Work out the finished part from the listing and answer in its coordinate system (mm). Face numbers are marked on the shaded views. A direction names the side the tool comes from. Give positions to 0.01 mm unless a question says otherwise; leave off trailing zeros. Write each loop counter-clockwise with the first axis right and the second up, starting at its lowest first coordinate (ties: lowest second). Pieces come first, ordered by that corner, then holes.
1) Determine the mould class of the marked faces 5, 6 and 7 for opening direction Z: pulls with the +Z half, pulls with the -Z half, needs draft (parallel to the pull), parting line crosses it, or undercut.
2) Find section B-B (y = 21). Determine the outline of the cut face in (x, z).
3) Given pin 1 Ø1 at (y, z) = (36, -4.5) entering from +X; pin 2 Ø12 at (y, z) = (18, 4) entering from -X; pin 3 Ø4 at (x, z) = (74.1, -1.7) entering from +Y; pin 4 Ø6.5 at (x, z) = (68.3, 21.5) entering from +Y, each flat-ended and moving along its own axis, determine where each tip first touches the part or whether it passes through.
4) Find section D-D (z = 16). Determine the outline of the cut face in (x, y).
5) A tool of negligible diameter and unlimited length cuts with its end or side. For the marked faces 1, 2, 3 and 4, from which of +Z, -Z, +X, -X, +Y, -Y can it reach the whole face along a straight path? Write none if from no direction.
6) Straight lines are drawn through the part: probe 1 along Z at (x, y) = (68, 23); probe 2 along Z at (x, y) = (-100, 9.75); probe 3 along Z at (x, y) = (-3.5, 8). For each, find the intervals that lie inside material, in ascending order.
7) Find section A-A (x = 74.1). Determine the outline of the cut face in (y, z), plus the area to 3 significant figures.
8) Find section C-C (x = 12). Determine the outline of the cut face in (y, z).
```python
from build123d import *
from build123d.topology import SkipClean

# Parameters (mm, degrees)
SKETCH1_W           = 195
SKETCH1_H           = 67
BOSS_EXTRUDE1_DEPTH = 50
CUT_EXTRUDE1_DEPTH  = 115.579666608
CUT_EXTRUDE2_DEPTH  = 129.433835106
CUT_EXTRUDE3_START  = -13
SKETCH4_W           = 3.612655346
SKETCH4_H           = 3
CUT_EXTRUDE3_DEPTH  = 13
SKETCH6_R           = 2.5
CUT_EXTRUDE4_DEPTH  = 115.579666608
SKETCH7_W           = 37
SKETCH7_H           = 35
CUT_EXTRUDE5_DEPTH  = 1.5
CUT_EXTRUDE6_DEPTH  = 18.5
SKETCH9_R           = 2.5
CUT_EXTRUDE7_DEPTH  = 25
BOSS_EXTRUDE2_START = 25
BOSS_EXTRUDE2_DEPTH = 25
BOSS_EXTRUDE3_DEPTH = 2


with BuildPart() as part:
    # Sketch1 → Boss-Extrude1 (new body)
    with BuildSketch(Plane(origin=(0, 0, 0), x_dir=(1, 0, 0), z_dir=(0, 1, 0))):
        Rectangle(SKETCH1_W, SKETCH1_H)
    extrude(amount=BOSS_EXTRUDE1_DEPTH)

    # Sketch2 → Cut-Extrude1 (cut, through all)
    with BuildSketch(Plane.XZ):
        with BuildLine():
            Line((97.5, -3.219751644), (97.5, 33.5))
            Line((97.5, 33.5), (88.5, 33.5))
            ThreePointArc((88.5, 33.5), (95.217186872, 15.683556008), (97.5, -3.219751644))
        make_face()
        with BuildLine():
            Line((97.5, -33.5), (97.5, -3.219751644))
            ThreePointArc((97.5, -3.219751644), (95.985558513, -18.65423771), (91.5, -33.5))
            Line((91.5, -33.5), (97.5, -33.5))
        make_face()
        with BuildLine():
            ThreePointArc((-88, -33.5), (-95.08607052, -15.861694529), (-97.5, 2.992884749))
            Line((-97.5, 2.992884749), (-97.5, -33.5))
            Line((-97.5, -33.5), (-88, -33.5))
        make_face()
        with BuildLine():
            ThreePointArc((-97.5, 2.992884749), (-95.856964648, 18.588830376), (-91, 33.5))
            Line((-91, 33.5), (-97.5, 33.5))
            Line((-97.5, 33.5), (-97.5, 2.992884749))
        make_face()
    extrude(amount=-CUT_EXTRUDE1_DEPTH, mode=Mode.SUBTRACT)

    # Sketch3 → Cut-Extrude2 (cut, through all)
    with BuildSketch(Plane(origin=(0, 0, 33.5), x_dir=(-1, 0, 0), z_dir=(0, 0, -1))):
        Polygon((63.2, 50), (63.2, 39.6), (40.2, 39.6), (40.2, 35.6), (-61.8, 35.6), (-61.8, 39.6), (-97.5, 39.6), (-97.5, 50), align=None)
    extrude(amount=CUT_EXTRUDE2_DEPTH, mode=Mode.SUBTRACT)

    # Sketch4 → Cut-Extrude3 (cut)
    with BuildSketch(Plane(origin=(0, 50, 0), x_dir=(1, 0, 0), z_dir=(0, 1, 0)).offset(CUT_EXTRUDE3_START)):
        with BuildLine():
            Line((-63.2, 30.5), (-63.2, 33.5))
            Line((-63.2, 33.5), (-88, 33.5))
            ThreePointArc((-88, 33.5), (-88.810680862, 32.008999469), (-89.587344654, 30.5))
            Line((-89.587344654, 30.5), (-63.2, 30.5))
        make_face()
        with Locations((-61.393672327, 32)):
            Rectangle(SKETCH4_W, SKETCH4_H)
        with BuildLine():
            Line((-63.2, -33.5), (-63.2, -30.5))
            Line((-63.2, -30.5), (-92.261692194, -30.5))
            ThreePointArc((-92.261692194, -30.5), (-91.647155152, -32.006859002), (-91, -33.5))
            Line((-91, -33.5), (-63.2, -33.5))
        make_face()
        with Locations((-61.393672327, -32)):
            Rectangle(SKETCH4_W, SKETCH4_H)
    extrude(amount=CUT_EXTRUDE3_DEPTH, mode=Mode.SUBTRACT)

    # Sketch6 → Cut-Extrude4 (cut, through all)
    with BuildSketch(Plane.XZ):
        with Locations(Location((-28.1, -9, 0), (0, 0, 270))):
            Circle(SKETCH6_R)
        with Locations(Location((-8.2, -8.3, 0), (0, 0, 270))):
            Circle(SKETCH6_R)
        with Locations(Location((-18.7, 8.7, 0), (0, 0, 270))):
            Circle(SKETCH6_R)
        with Locations(Location((-76.2, 22, 0), (0, 0, 270))):
            Circle(SKETCH6_R)
        with Locations(Location((-78.2, 0.1, 0), (0, 0, 270))):
            Circle(SKETCH6_R)
        with Locations(Location((-73.2, -22.3, 0), (0, 0, 270))):
            Circle(SKETCH6_R)
        with Locations(Location((65.3, -20, 0), (0, 0, 270))):
            Circle(SKETCH6_R)
        with Locations(Location((74.1, -1.7, 0), (0, 0, 270))):
            Circle(SKETCH6_R)
        with Locations(Location((68.3, 21.5, 0), (0, 0, 270))):
            Circle(SKETCH6_R)
    extrude(amount=-CUT_EXTRUDE4_DEPTH, mode=Mode.SUBTRACT)

    # Sketch7 → Cut-Extrude5 (cut)
    with BuildSketch(Plane(origin=(0, 35.6, 0), x_dir=(1, 0, 0), z_dir=(0, 1, 0))):
        with Locations((5.3, -16)):
            Rectangle(SKETCH7_W, SKETCH7_H)
    extrude(amount=-CUT_EXTRUDE5_DEPTH, mode=Mode.SUBTRACT)

    # Sketch8 → Cut-Extrude6 (cut)
    with BuildSketch(Plane(origin=(0, 50, 0), x_dir=(1, 0, 0), z_dir=(0, 1, 0))):
        with BuildLine():
            Line((37.096152423, 33.5), (31.9, 33.5))
            Line((31.9, 33.5), (31.9, 30.5))
            ThreePointArc((31.9, 30.5), (34.9, 31.303847577), (37.096152423, 33.5))
        make_face()
        with BuildLine():
            Line((31.9, 33.5), (26.703847577, 33.5))
            ThreePointArc((26.703847577, 33.5), (28.9, 31.303847577), (31.9, 30.5))
            Line((31.9, 30.5), (31.9, 33.5))
        make_face()
    extrude(amount=-CUT_EXTRUDE6_DEPTH, mode=Mode.SUBTRACT)

    # Sketch9 → Cut-Extrude7 (cut)
    with BuildSketch(Plane.XZ):
        with BuildLine():
            Line((-2.396551724, 28.5), (-81.585940529, 28.5))
            ThreePointArc((-81.585940529, 28.5), (-82.773060502, 28.814676047), (-83.648434047, 29.676067945))
            ThreePointArc((-83.648434047, 29.676067945), (-85.016854467, 31.683550399), (-86.630258043, 33.5))
            Line((-86.630258043, 33.5), (-91, 33.5))
            ThreePointArc((-91, 33.5), (-96.041663789, 17.695271398), (-97.477752055, 1.168158207))
            ThreePointArc((-97.477752055, 1.168158207), (-95.332095511, 1.5823273), (-93.248186912, 2.240128941))
            ThreePointArc((-93.248186912, 2.240128941), (-90, -7e-09), (-93.248186926, -2.240128936))
            ThreePointArc((-93.248186926, -2.240128936), (-95.286014537, -1.594067776), (-97.383519589, -1.181019415))
            ThreePointArc((-97.383519589, -1.181019415), (-94.531917422, -17.874782597), (-88, -33.5))
            Line((-88, -33.5), (-86.630258043, -33.5))
            ThreePointArc((-86.630258043, -33.5), (-85.016854382, -31.683550291), (-83.648433906, -29.676067708))
            ThreePointArc((-83.648433906, -29.676067708), (-82.773060382, -28.814675978), (-81.585940529, -28.5))
            Line((-81.585940529, -28.5), (-2.396551708, -28.5))
            ThreePointArc((-2.396551708, -28.5), (-0.701933743, -27.798066246), (0, -26.103448276))
            Line((0, -26.103448276), (0, -9.896551726))
            ThreePointArc((0, -9.896551726), (0.701933748, -8.201933749), (2.396551724, -7.5))
            Line((2.396551724, -7.5), (97.384558849, -7.5))
            ThreePointArc((97.384558849, -7.5), (97.434108416, 0.014482123), (96.773110049, 7.5))
            Line((96.773110049, 7.5), (2.396551724, 7.5))
            ThreePointArc((2.396551724, 7.5), (0.70193375, 8.201933747), (0, 9.896551721))
            Line((0, 9.896551721), (0, 26.103448276))
            ThreePointArc((0, 26.103448276), (-0.701933749, 27.798066251), (-2.396551724, 28.5))
        make_face()
        with Locations(Location((-73.2, -22.3, 0), (0, 0, 270))):
            Circle(SKETCH9_R, mode=Mode.SUBTRACT)
        with Locations(Location((-78.2, 0.1, 0), (0, 0, 270))):
            Circle(SKETCH9_R, mode=Mode.SUBTRACT)
        with Locations(Location((-28.1, -9, 0), (0, 0, 270))):
            Circle(SKETCH9_R, mode=Mode.SUBTRACT)
        with Locations(Location((-8.2, -8.3, 0), (0, 0, 270))):
            Circle(SKETCH9_R, mode=Mode.SUBTRACT)
        with Locations(Location((-76.2, 22, 0), (0, 0, 270))):
            Circle(SKETCH9_R, mode=Mode.SUBTRACT)
        with Locations(Location((-18.7, 8.7, 0), (0, 0, 270))):
            Circle(SKETCH9_R, mode=Mode.SUBTRACT)
        with Locations(Location((74.1, -1.7, 0), (0, 0, 270))):
            Circle(SKETCH9_R, mode=Mode.SUBTRACT)
    extrude(amount=-CUT_EXTRUDE7_DEPTH, mode=Mode.SUBTRACT)

    # Sketch10 → Boss-Extrude2 (add)
    with SkipClean():  # the faces are left unmerged after this step: merging them gives an invalid solid
        with BuildSketch(Plane.XZ.offset(-25).offset(BOSS_EXTRUDE2_START)):
            with BuildLine():
                ThreePointArc((-97.477752055, 1.168158207), (-118.013212767, 26.043522633), (-86.630258043, 33.5))
                Line((-86.630258043, 33.5), (88.5, 33.5))
                ThreePointArc((88.5, 33.5), (85.908246666, 38.091048485), (83.017561959, 42.5))
                Line((83.017561959, 42.5), (-119.771431792, 42.5))
                ThreePointArc((-119.771431792, 42.5), (-127.448858613, -0.281382159), (-117.115521807, -42.5))
                Line((-117.115521807, -42.5), (87.104231658, -42.5))
                ThreePointArc((87.104231658, -42.5), (89.444159442, -38.069376757), (91.5, -33.5))
                Line((91.5, -33.5), (-86.630258043, -33.5))
                ThreePointArc((-86.630258043, -33.5), (-118.028282029, -25.998420382), (-97.383519589, -1.181019415))
                ThreePointArc((-97.383519589, -1.181019415), (-97.43986106, -0.006800655), (-97.477752055, 1.168158207))
            make_face()
        extrude(amount=-BOSS_EXTRUDE2_DEPTH)

    # Sketch11 → Boss-Extrude3 (add)
    with SkipClean():  # the faces are left unmerged after this step: merging them gives an invalid solid
        with BuildSketch(Plane(origin=(0, 25, 0), x_dir=(1, 0, 0), z_dir=(0, 1, 0))):
            with BuildLine():
                ThreePointArc((83.017561959, -42.5), (85.908246666, -38.091048485), (88.5, -33.5))
                Line((88.5, -33.5), (-91, -33.5))
                ThreePointArc((-91, -33.5), (-97.425088146, 0.354854693), (-88, 33.5))
                Line((-88, 33.5), (91.5, 33.5))
                ThreePointArc((91.5, 33.5), (89.444159442, 38.069376757), (87.104231658, 42.5))
                Line((87.104231658, 42.5), (-117.115521807, 42.5))
                ThreePointArc((-117.115521807, 42.5), (-127.448858613, 0.281382159), (-119.771431792, -42.5))
                Line((-119.771431792, -42.5), (83.017561959, -42.5))
            make_face()
        extrude(amount=BOSS_EXTRUDE3_DEPTH)


solid = part.part
```
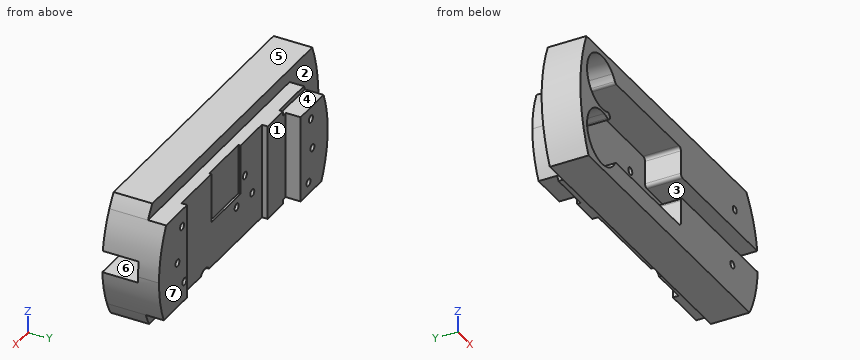
Results:
1. face 5: pulls with the +Z half
1. face 6: undercut
1. face 7: needs draft
2. outline: (-119.77, 42.5) arc R104.84 ccw to (-117.12, -42.5) - (87.1, -42.5) arc R79.41 ccw to (97.38, -7.5) - (2.4, -7.5) arc R2.4 ccw to (0, -9.9) - (0, -26.1) arc R2.4 cw to (-2.4, -28.5) - (-81.59, -28.5) arc R2.4 ccw to (-83.65, -29.68) arc R19 cw (long way) to (-93.25, -2.24) arc R2.4 ccw (long way) to (-93.25, 2.24) arc R19 cw (long way) to (-83.65, 29.68) arc R2.4 ccw to (-81.59, 28.5) - (-2.4, 28.5) arc R2.4 cw to (0, 26.1) - (0, 9.9) arc R2.4 ccw to (2.4, 7.5) - (96.77, 7.5) arc R79.41 ccw to (83.02, 42.5) - close; hole circle Ø5 at (65.3, -20); hole circle Ø5 at (68.3, 21.5)
3. pin 1: stops at x = 97.5
3. pin 2: stops at x = -127.5
3. pin 3: passes through
3. pin 4: stops at y = 39.6
4. outline: (-126.69, 0) - (-118.57, 0) - (-118.57, 25) - (0, 25) - (0, 0) - (95.14, 0) - (95.14, 39.6) - (61.8, 39.6) - (61.8, 35.6) - (23.8, 35.6) - (23.8, 34.1) - (-13.2, 34.1) - (-13.2, 35.6) - (-40.2, 35.6) - (-40.2, 39.6) - (-63.2, 39.6) - (-63.2, 50) - (-96.36, 50) - (-96.36, 27) - (-126.69, 27) - close
5. face 1: +Z, -Z, +X, +Y
5. face 2: -X, +Y
5. face 3: +X, -Y
5. face 4: +Z, -X, +Y
6. probe 1: z = -42.5 to -7.5, 7.5 to 19.02, 23.98 to 42.5
6. probe 2: z = -42.5 to -39, -1 to 1, 39 to 42.5
6. probe 3: z = -42.5 to -28.5, 28.5 to 42.5
7. outline: (0, -42.5) - (27, -42.5) - (27, -33.5) - (39.6, -33.5) - (39.6, -4.2) - (25, -4.2) - (25, -7.5) - (0, -7.5) - close; (0, 7.5) - (25, 7.5) - (25, 0.8) - (39.6, 0.8) - (39.6, 33.5) - (27, 33.5) - (27, 42.5) - (0, 42.5) - close
7. area: 2,690 mm2
8. outline: (0, -42.5) - (27, -42.5) - (27, -33.5) - (35.6, -33.5) - (35.6, -1.5) - (34.1, -1.5) - (34.1, 33.5) - (27, 33.5) - (27, 42.5) - (0, 42.5) - (0, 7.5) - (25, 7.5) - (25, -7.5) - (0, -7.5) - close
